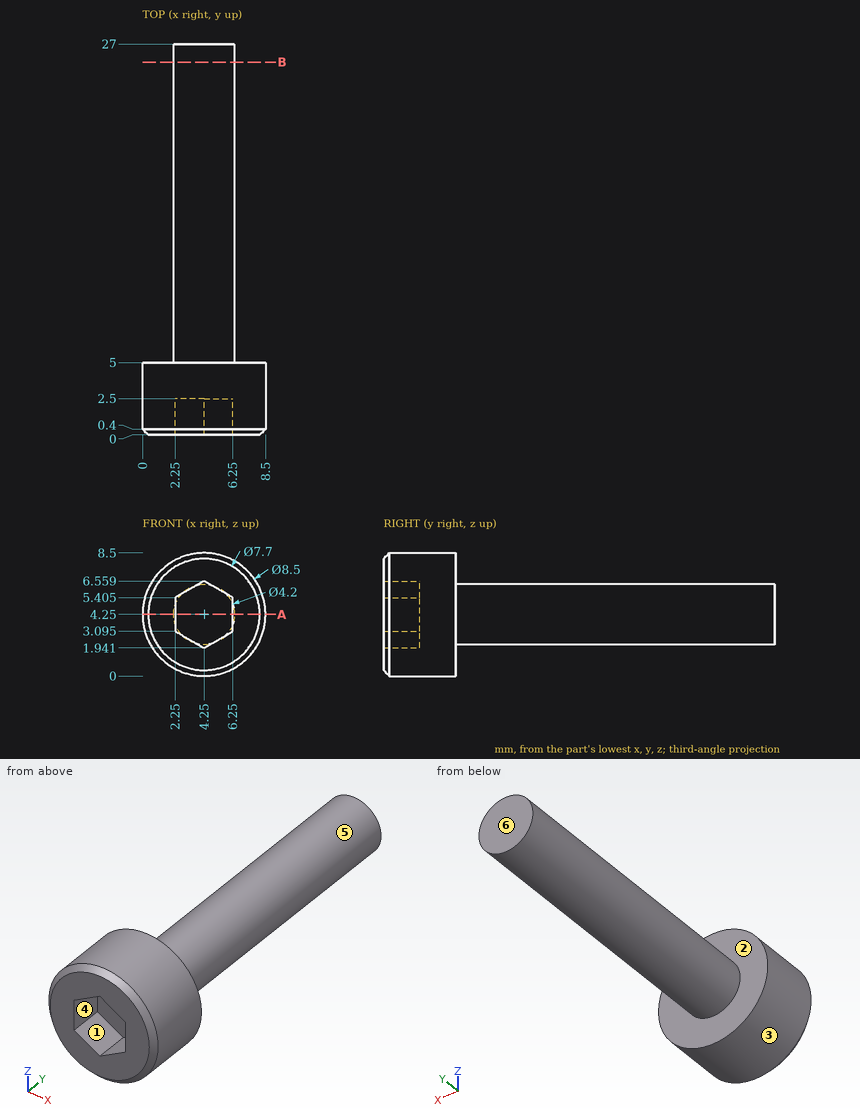
Check sheet for the drawn part. Datum: minimum x, y, z corner. Units: mm. A direction names the side the tool comes from. Coordinates: 2 decimals unless noted, no trailing zeros. Loops run counter-clockwise (first coordinate to the right, second up) from the corner with the lowest first, then second, coordinate; pieces in that order, holes last. Notation, with made-up numbers: M 40,34.5 L 66,34.5 A19 ccw 66,52.5 Z; hole C 5,10 d2. An arc over 180 degrees is marked long. Answer as a JSON object with one key per item and string values.
1. Depth check by flat-ended pin: P1, Ø2, axis at x = 4, z = 4.5, coming from the -Y side; P2, Ø1.5, axis at y = 18, z = 2, coming from the -X side; P3, Ø1, axis at x = 3, y = 13.5, coming from the +Z side. Enter the tip coordinate at first touch or a pass-through.
Outcome:
{"P1": "y = 2.5", "P2": "x = 2.78", "P3": "z = 6.21"}
2. Sectioned sample at B-B on y = 25.75. Record the cut outline in (x, z).
Outcome:
{"outline": "C 4.25,4.25 d4.2"}
3. Release check for a two-part mould opening along X. For the marked faces 4, 5 and 6 record: pulls with the +X half, pulls with the -X half, needs draft (parallel to the pull), parting line crosses it, or undercut.
Outcome:
{"face 4": "undercut", "face 5": "parting line crosses it", "face 6": "needs draft"}
4. Sectioned sample at A-A on z = 4.25. Record the cut outline in (x, y).
Outcome:
{"outline": "M 0,0.4 L 0.4,0 L 2.25,0 L 2.25,2.5 L 6.25,2.5 L 6.25,0 L 8.1,0 L 8.5,0.4 L 8.5,5 L 6.35,5 L 6.35,27 L 2.15,27 L 2.15,5 L 0,5 Z"}
5. Access from +Z, -Z, +X, -X, +Y, -Y to the whole of each face (thin tool, end or side, straight path). Record for the marked faces 1, 2 and 3.
Outcome:
{"face 1": "-Y", "face 2": "+Y", "face 3": "+Y, -Y"}
6. Scan lines: L1, parallel to Z at x = 6, y = 25; L2, parallel to Y at x = 3.25, z = 2.25. Record each from-to range of solid material in increasing order. Write a range as from..to.
Outcome:
{"L1": "3.09..5.41", "L2": "0..5"}
